Here's how the part is built. I have some questions about the finished solid (model axes, mm). Face numbers are marked on the shaded views. Round coordinates to 2 decimals unless told otherwise and drop trailing zeros. Order: outer loops, then holes, each group sorted by start corner. A loop starts at its lowest first (then second) coordinate and runs counter-clockwise, first axis right, second up. Notation, with made-up numbers: (72, 88.25) - (91, 88.25) arc R25 ccw to (91, 115.25) - close; hole circle Ø6 at (-33, 78.5). An arc over 180 degrees is marked (long way). One line per item, written item: value.
from build123d import *

# Parameters (mm, degrees)
SKETCH_W        = 71
SKETCH_H        = 190
PAD_DEPTH       = 3
SKETCH001_R     = 1.5
SKETCH001_W     = 14
SKETCH001_H     = 14
SKETCH001_W_2   = 2
SKETCH001_H_2   = 108
POCKET_DEPTH    = 3
SKETCH002_W     = 71
SKETCH002_H     = 3
PAD001_DEPTH    = 60
FILLET_R        = 5
SKETCH003_W     = 20
SKETCH003_H     = 20
POCKET001_DEPTH = 2
SKETCH004_W     = 50
SKETCH004_H     = 45
POCKET002_DEPTH = 200


with BuildPart() as part:
    # Sketch → Pad (new body)
    with BuildSketch(Plane.XY):
        Rectangle(SKETCH_W, SKETCH_H)
    extrude(amount=PAD_DEPTH)

    # Sketch001 (on Face6 of Pad) → Pocket (cut)
    with BuildSketch(Plane.XY.offset(3)):
        with Locations((-15.5, 70)):
            Circle(SKETCH001_R)
        with Locations((-15.5, -50)):
            Circle(SKETCH001_R)
        with Locations((15.5, 70)):
            Circle(SKETCH001_R)
        with Locations((15.5, -50)):
            Circle(SKETCH001_R)
        with Locations((-15.5, -72)):
            Rectangle(SKETCH001_W, SKETCH001_H)
        with Locations((-15.5, 10)):
            Rectangle(SKETCH001_W_2, SKETCH001_H_2)
        with Locations((15.5, -72)):
            Rectangle(SKETCH001_W, SKETCH001_H)
        with Locations((15.5, 10)):
            Rectangle(SKETCH001_W_2, SKETCH001_H_2)
    extrude(amount=-POCKET_DEPTH, mode=Mode.SUBTRACT)

    # Sketch002 (on Face5 of Pocket) → Pad001 (join)
    with BuildSketch(Plane.XY.offset(3)):
        with Locations((0, 93.5)):
            Rectangle(SKETCH002_W, SKETCH002_H)
        with Locations((0, -93.5)):
            Rectangle(SKETCH002_W, SKETCH002_H)
    extrude(amount=PAD001_DEPTH)

    # Fillet
    fillet_edges = [part.edges().sort_by_distance(p)[0] for p in [
        (0, 92, 3),
        (0, -92, 3),
    ]]
    fillet(fillet_edges, radius=FILLET_R)

    # Sketch003 (on Face2 of Fillet) → Pocket001 (cut)
    with BuildSketch(Plane.XY.offset(3)):
        with Locations((-15.5, -72)):
            Rectangle(SKETCH003_W, SKETCH003_H)
        with Locations((15.5, -72)):
            Rectangle(SKETCH003_W, SKETCH003_H)
    extrude(amount=-POCKET001_DEPTH, mode=Mode.SUBTRACT)

    # Sketch004 (on Face33 of Pocket001) → Pocket002 (cut)
    with BuildSketch(Plane.XZ.offset(95)):
        with Locations((-0.5, 30.5)):
            Rectangle(SKETCH004_W, SKETCH004_H)
    extrude(amount=-POCKET002_DEPTH, mode=Mode.SUBTRACT)


solid = part.part
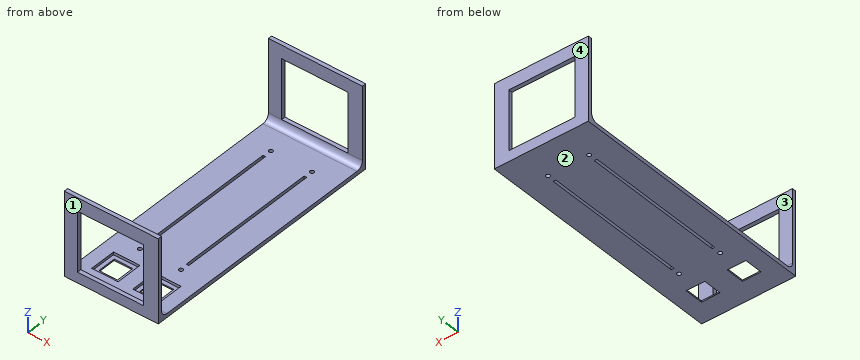
Q1. If we section it at B-B, the plane x = -3: Please give me the cut outline in (y, z).
Results list:
outline: (-95, 0) - (95, 0) - (95, 8) - (92, 8) arc R5 cw to (87, 3) - (-87, 3) arc R5 cw to (-92, 8) - (-95, 8) - close; (-95, 53) - (-92, 53) - (-92, 63) - (-95, 63) - close; (92, 53) - (95, 53) - (95, 63) - (92, 63) - close
Q2. We'd pull the mould along Y, two halves only. Please class the marked faces 1, 2, 3 and 4: released by +Y, released by -Y, zero draft, split by the parting line, or undercut.
Results list:
face 1: released by -Y
face 2: zero draft
face 3: undercut
face 4: released by +Y
Q3. Will this pin go through, and if not, where does the flat tip stop? pin 1 (3 mm diameter, centred on x = 14.5, y = -42, fed in from +Z).
Results list:
pin 1: z = 3
Q4. If we section it at C-C, the plane x = 30: Please give me the cut outline in (y, z), then the cut area to 3 significant figures.
Results list:
outline: (-95, 0) - (95, 0) - (95, 63) - (92, 63) - (92, 8) arc R5 cw to (87, 3) - (-87, 3) arc R5 cw to (-92, 8) - (-92, 63) - (-95, 63) - close
area: 941 mm²
Q5. If we section it at A-A, the plane z = 50.5: Please give me the cut outline in (x, y), then the cut area to 3 significant figures.
Results list:
outline: (-35.5, -95) - (-25.5, -95) - (-25.5, -92) - (-35.5, -92) - close; (-35.5, 92) - (-25.5, 92) - (-25.5, 95) - (-35.5, 95) - close; (24.5, -95) - (35.5, -95) - (35.5, -92) - (24.5, -92) - close; (24.5, 92) - (35.5, 92) - (35.5, 95) - (24.5, 95) - close
area: 126 mm²
Q6. If we section it at D-D, the plane y = -46: Please give me the cut outline in (x, z), then the cut area to 3 significant figures.
Results list:
outline: (-35.5, 0) - (35.5, 0) - (35.5, 3) - (-35.5, 3) - close
area: 213 mm²
Q7. If I drill on line 1 along Y through (x, z) = (-15.5, 1.35); line 2 along X through (y, z) = (70, 0.6); line 3 along Y through (x, z) = (-30, 21.5), over which ranges is the centre line in solid material (lowest first)?
Results list:
line 1: -95 to -82, -62 to -51.5, -48.5 to -44, 64 to 68.5, 71.5 to 95
line 2: -35.5 to -17, -14 to 14, 17 to 35.5
line 3: -95 to -92, 92 to 95
